The listing builds one solid part. Answer for the finished solid, in the listing's coordinates (mm). A direction names the side the tool comes from. Coordinates: 2 decimals unless noted, no trailing zeros. Order: outer loops, then holes, each group sorted by start corner. A loop starts at its lowest first (then second) coordinate and runs counter-clockwise, first axis right, second up. Notation, with made-up numbers: M -1.5,-10 L 42.5,-10 A8 ccw 42.5,-6 Z; hole C 51.25,-15.75 d8. An arc over 180 degrees is marked long. One line per item, written item: value. Start each with the question number.
Q1. The part is cut by section B-B on z = 4.25. Give the number of separate pieces and of enclosed holes in the cut face, then the cut area to 3 significant figures.
Q2. Determine the mould class of faces 4 (the flat face through (0, 8, 5)), 5 (the flat face through (3, 18, 5)), 6 (the flat face through (16, -1, 5)) for opening direction Y: pulls with the +Y half, pulls with the -Y half, needs draft (parallel to the pull), parting line crosses it, or undercut.
Q3. The part is cut by section D-D on x = 5.5. Give the vertices of the cut face in (y, z).
Q4. Each of these flat-tipped pins is pushed along its axis until it touches: pin 1 Ø2 at (x, z) = (21, 1) entering from +Y; pin 2 Ø0.8 at (x, y) = (21.5, -1) entering from -Z; pin 3 Ø2 at (x, z) = (34, 5.5) entering from +Y; pin 4 Ø4 at (y, z) = (6.5, 3.5) entering from -X. Where does it stop, or does it pass through?
Q5. Straight lines are drawn through the part: line 1 along Y through (x, z) = (2.75, 5.75); line 2 along Y through (x, z) = (2.75, 7.25); line 3 along Y through (x, z) = (32, 2). For each, find the intervals that lie inside material, in ascending order. Write a range as [from, to].
Q6. For faces 1 (the flat face through (33, 11.25, 5)), 2 (the flat face through (4.3, 17.7, 2.5)), 3 (the cylindrical face through (0.9, 15.14, 4.82)), determine the directions among +Z, -Z, +X, -X, +Y, -Y from which every point of the face is accessible in a straight line to the end or side of a thin tool.
Q7. The part is cut by section A-A on x = 30.5. Give the vertices of the cut face in (y, z), then the cut area to 3 significant figures.
Q8. The part is cut by section C-C on y = 9.75. Give the vertices of the cut face in (x, z), then the cut area to 3 significant figures.
Autodesk Inventor part; units mm, degrees
ref_plane "YZ Plane" through (0, 0, 0) normal (1, 0, 0) x (0, 1, 0)
ref_plane "XZ Plane" through (0, 0, 0) normal (0, 1, 0) x (-1, 0, 0)
ref_plane "XY Plane" through (0, 0, 0) normal (0, 0, 1) x (1, 0, 0)
sketch "スケッチ1" plane through (0, 0, 0) normal (0, 0, 1) x (1, 0, 0)
  line L0 (0, 0) -> (28, 0)
  line L1 (28, 0) -> (28, 16)
  line L2 (28, 16) -> (0, 16)
  line L3 (0, 16) -> (0, 0)
  line L4 (0, 11.25) -> (0, 4.75)
  dimension "d0" = 28
  dimension "d1" = 16
  dimension "d2" = 6.5
  dimension "d3" = 4.75
extrude "押し出し1" add sketch "スケッチ1" along normal blind 9.5
sketch "スケッチ2" plane through (28, 0, 0) normal (1, 0, 0) x (0, 0, -1)
  line L0 (0, 16) -> (0, 0)
  line L1 (0, 11.25) -> (0, 4.75)
  line L2 (0, 16) -> (-9.5, 16)
  line L3 (-8, 16) -> (-1.5, 16)
  line L4 (-8, 11.25) -> (-1.5, 11.25)
  line L5 (-1.5, 11.25) -> (-1.5, 10.75)
  line L6 (-1.5, 10.75) -> (-8, 10.75)
  line L7 (-8, 10.75) -> (-8, 11.25)
  line L8 (-8, 4.75) -> (-1.5, 4.75)
  line L9 (-1.5, 4.75) -> (-1.5, 5.25)
  line L10 (-1.5, 5.25) -> (-8, 5.25)
  line L11 (-8, 5.25) -> (-8, 4.75)
  dimension "d6" = 6.5
  dimension "d7" = 4.75
  dimension "d8" = 6.5
  dimension "d9" = 1.5
  dimension "d10" = 0.5
  dimension "d11" = 0.5
extrude "押し出し2" add sketch "スケッチ2" along normal blind 10
sketch "スケッチ3" plane through (0, 16, 0) normal (0, 1, 0) x (1, 0, 0)
  line L0 (0, -9.5) -> (28, -9.5)
  line L1 (17, -9.5) -> (17, 0)
  line L2 (28, 0) -> (28, -9.5)
  line L3 (17, -7) -> (17, -2.5)
  line L4 (17, -7) -> (16.5, -7)
  line L5 (16.5, -7) -> (16.5, -2.5)
  line L6 (16.5, -2.5) -> (17, -2.5)
  line L7 (17, -2.5) -> (17, -7)
  point P0 (0, 0)
  dimension "d14" = 11
  dimension "d15" = 4.5
  dimension "d16" = 2.5
  dimension "d17" = 0.5
extrude "押し出し3" add sketch "スケッチ3" along normal blind 2
sketch "スケッチ4" plane through (16.5, 16, 2.5) normal (-1, 0, 0) x (0, 0, 1)
  line L0 (0, 2) -> (4.5, 2)
  line L1 (4.5, 0) -> (4.5, 2)
  line L2 (0, 2) -> (4.5, 2)
  line L3 (4.5, 2) -> (4.5, 1.5)
  line L4 (4.5, 1.5) -> (0, 1.5)
  line L5 (0, 1.5) -> (0, 2)
  point P0 (-2.5, -16)
  dimension "d20" = 0.5
extrude "押し出し4" add sketch "スケッチ4" along normal blind 27
sketch "スケッチ5" plane through (0, 0, 0) normal (0, -1, 0) x (1, 0, 0)
  line L0 (28, 9.5) -> (0, 9.5)
  line L1 (28, 0) -> (0, 0)
  line L2 (15.5, 9.5) -> (15.5, 0)
  line L3 (0, 0) -> (0, 9.5)
  line L4 (15.5, 8) -> (15.5, 1.5)
  line L5 (15.5, 8) -> (16, 8)
  line L6 (16, 8) -> (16, 1.5)
  line L7 (16, 1.5) -> (15.5, 1.5)
  line L8 (15.5, 1.5) -> (15.5, 8)
  dimension "d23" = 15.5
  dimension "d24" = 6.5
  dimension "d25" = 1.5
  dimension "d26" = 0.5
extrude "押し出し5" add sketch "スケッチ5" along normal blind 2.5 contours L5 L6 L7 L2
sketch "スケッチ6" plane through (16, 0, 8) normal (1, 0, 0) x (0, 0, -1)
  line L0 (0, -2.5) -> (6.5, -2.5)
  line L1 (0, 0) -> (0, -2.5)
  line L2 (6.5, -2.5) -> (0, -2.5)
  line L3 (0, -2.5) -> (0, -2)
  line L4 (0, -2) -> (6.5, -2)
  line L5 (6.5, -2) -> (6.5, -2.5)
  point P0 (8, 0)
  dimension "d29" = 0.5
extrude "押し出し6" add sketch "スケッチ6" along normal blind 9
sketch "スケッチ7" plane through (0, 0, 0) normal (0, 0, -1) x (-1, 0, 0)
  line L0 (0, 16) -> (0, 0)
  line L1 (-28, 16) -> (0, 16)
  line L2 (-28, 0) -> (-28, 16)
  line L3 (0, 0) -> (-28, 0)
  point P0 (-2.75, 2.75)
  point P1 (-25.25, 13.25)
  dimension "d32" = 2.75
  dimension "d34" = 2.75
  dimension "d35" = 13.25
  dimension "d43" = 2.75
hole "穴1" at (2.75, 2.75, 0) at (25.25, 13.25, 0) direction (0, 0, 1) diameter 3.5 end through all
fillet "フィレット1" radius 3 4 edges at (0, 0, 4.75) (0, 16, 4.75) (28, 16, 4.75) (28, 0, 4.75)
equation "\"d33\" = d32"
properties part number "switch_V_152_1A5_KM"
Output:
1. separate pieces: 1
1. enclosed holes: 2
1. area: 451 mm^2
2. face 4: needs draft
2. face 5: pulls with the +Y half
2. face 6: undercut
3. outline: M 0,0 L 16,0 L 16,9.5 L 0,9.5 Z; M 17.5,2.5 L 18,2.5 L 18,7 L 17.5,7 Z
4. pin 1: stops at y = 16
4. pin 2: passes through
4. pin 3: stops at y = 11.25
4. pin 4: stops at x = 0
5. line 1: y = [0.01, 1], [4.5, 15.99], [17.5, 18]
5. line 2: y = [0.01, 1], [4.5, 15.99]
5. line 3: y = [4.75, 5.25], [10.75, 11.25]
6. face 1: +Z, -Z, +X, +Y
6. face 2: -Z, +X, -X, +Y
6. face 3: +Z, -Z, -X
7. outline: M 4.75,1.5 L 5.25,1.5 L 5.25,8 L 4.75,8 Z; M 10.75,1.5 L 11.25,1.5 L 11.25,8 L 10.75,8 Z
7. area: 6.50 mm^2
8. outline: M 0,0 L 28,0 L 28,9.5 L 0,9.5 Z
8. area: 266 mm^2
